Input: part model. Units: mm. Frame: model coordinates. Give positions to 0.01 mm unless a question says otherwise; leave off trailing zeros. Write each loop counter-clockwise with the first axis right and the second up, starting at its lowest first coordinate (ties: lowest second). Pieces come first, ordered by that corner, then holes. Notation, with made-up numbers: (64.5, 59.25) - (96.5, 59.25) arc R9 ccw to (96.5, 67.25) - close; hole circle Ø8 at (75.5, 16.5). An arc over 180 degrees is marked (long way). Answer as CSV lines item,"result". Start each with the question number.
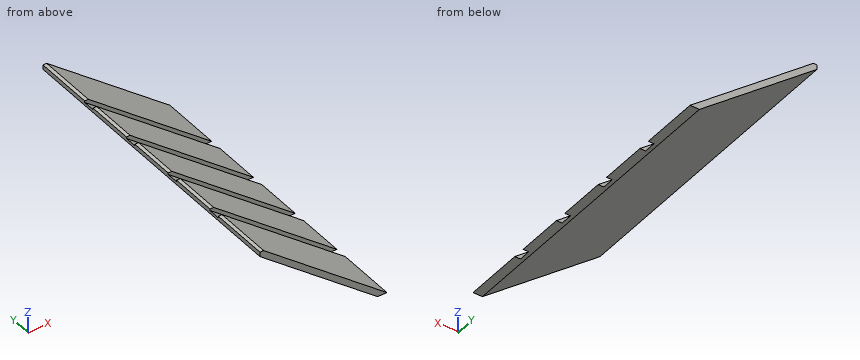
from build123d import *

# Parameters (mm, degrees)
F1_DEPTH = 330.2
F2_W     = 228.6
F2_H     = 12.7
F3_DEPTH = 3.81


with BuildPart() as f1:
    # F0 (on Front) → F1 (new body)
    with BuildSketch(Plane.XZ):
        Polygon((0, 106.55851694), (0, 101.6), (127, 0), (137.1649597269, 0), (3.966813552, 106.55851694), align=None)
    extrude(amount=F1_DEPTH)

    # F2 (on face) → F3 (cut)
    with BuildSketch(Plane(origin=(53.5277891617, 0, 66.9097364522), x_dir=(0.7808688094, 0, -0.6246950476), z_dir=(0.6246950476, 0, 0.7808688094))):
        with Locations((21.8194109839, -260.35)):
            Rectangle(F2_W, F2_H)
        with Locations((21.8194109839, -196.85)):
            Rectangle(F2_W, F2_H)
        with Locations((21.8194109839, -133.35)):
            Rectangle(F2_W, F2_H)
        with Locations((21.8194109839, -69.85)):
            Rectangle(F2_W, F2_H)
    extrude(amount=-F3_DEPTH, mode=Mode.SUBTRACT)


solid = f1.part
1) Contact query for flat-ended pins moving along their axis: P1, Ø1.5, axis at y = -83, z = 28.5, coming from the -X side; P2, Ø2, axis at x = 24.5, y = -169.5, coming from the -Z side; P3, Ø2, axis at y = -275.5, z = 87, coming from the -X side. Output: stop coordinate, or through.
2) Cut plane A-A on z = 73. Output: boundary loops of the cut face in (x, y), and give its area (3 significant figures).
3) Cut plane B-B on y = -37. Output: boundary loops of the cut face in (x, z), and give its area (3 significant figures).
4) Cut plane C-C on x = 76. Output: boundary loops of the cut face in (y, z).
5) Material intervals for line 1 (Z direction, x = 107, y = -262.5); line 2 (Z direction, x = 106.5, y = -233); line 3 (X direction, y = -192, z = 93), sorted ascending. Write a range as from..to.
Numbers:
1,P1,"stops at x = 90.44"
1,P2,"stops at z = 81.2"
1,P3,"stops at x = 17"
2,outline,"(35.75, -330.2) - (45.91, -330.2) - (45.91, -266.7) - (39.82, -266.7) - (39.82, -254) - (45.91, -254) - (45.91, -203.2) - (39.82, -203.2) - (39.82, -190.5) - (45.91, -190.5) - (45.91, -139.7) - (39.82, -139.7) - (39.82, -127) - (45.91, -127) - (45.91, -76.2) - (39.82, -76.2) - (39.82, -63.5) - (45.91, -63.5) - (45.91, 0) - (35.75, 0) - close"
2,area,"3,050 mm²"
3,outline,"(0, 101.6) - (127, 0) - (137.16, 0) - (3.97, 106.56) - (0, 106.56) - close"
3,area,"1,070 mm²"
4,outline,"(-330.2, 40.8) - (0, 40.8) - (0, 48.93) - (-63.5, 48.93) - (-63.5, 44.05) - (-76.2, 44.05) - (-76.2, 48.93) - (-127, 48.93) - (-127, 44.05) - (-139.7, 44.05) - (-139.7, 48.93) - (-190.5, 48.93) - (-190.5, 44.05) - (-203.2, 44.05) - (-203.2, 48.93) - (-254, 48.93) - (-254, 44.05) - (-266.7, 44.05) - (-266.7, 48.93) - (-330.2, 48.93) - close"
5,line 1,"z = 16..19.25"
5,line 2,"z = 16.4..24.53"
5,line 3,"x = 10.75..14.82"
